Geometry: final body of the model. Coordinates: model frame, mm. Face numbers are marked on the shaded views. A direction names the side the tool comes from. Coordinates: 2 decimals unless noted, no trailing zeros. Loops run counter-clockwise (first coordinate to the right, second up) from the corner with the lowest first, then second, coordinate; pieces in that order, holes last. Notation, with made-up numbers: (45.25, 39.5) -> (72.25, 39.5) arc R10 cw to (72.25, 47.5) -> close; hole circle Ø1 at (11.5, 46). An arc over 180 degrees is marked (long way). One line per item, written item: value. Start each with the question number.
Item 1: Section query B-B on x = 44. Return loops of the section in (y, z).
Item 2: Contact query for flat-ended pins moving along their axis: pin 1 Ø5 at (y, z) = (-2, -19.5) entering from -X; pin 2 Ø10 at (x, z) = (20, 16.5) entering from -Y; pin 3 Ø3 at (x, z) = (-46.5, 14.5) entering from -Y; pin 4 Ø10 at (x, y) = (58, -6.5) entering from -Z. Output: stop coordinate, or through.
Item 3: Section query C-C on x = -35. Return loops of the section in (y, z).
Item 4: Ray query, probe 1 along Z at (x, y) = (52.5, -1); probe 2 along X at (y, z) = (-19.5, -15); probe 3 along Y at (x, z) = (-54, 0.5). Return the intervals inside material, ascending. Write a range as from..to.
Item 5: Mould query, pull axis Z, two halves, no side actions, for the marked faces 3, 4 and 5. Classes: +Z half, -Z half, draft (parallel to the pull), parting line (faces both ways), or undercut.
Item 6: Section query A-A on z = 0. Return loops of the section in (x, y).
Item 7: Set-up query: the marked faces 1 and 2. Return all of +Z, -Z, +X, -X, +Y, -Y with unobstructed straight access to the full face (end or side cutting, diameter ignored); none if empty.
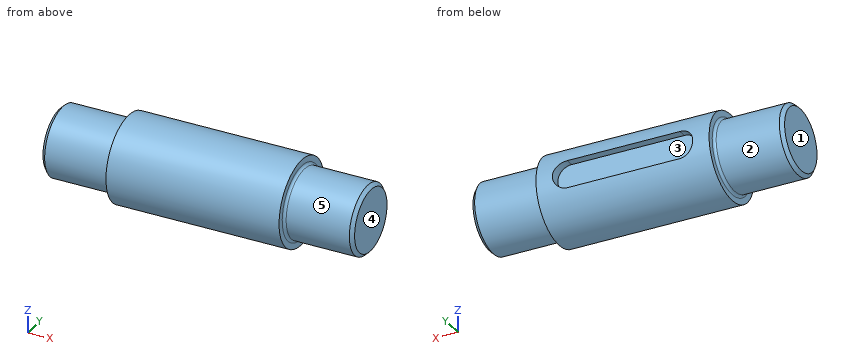
from build123d import *

# Parameters (mm, degrees)
CHANFREIN1_SIZE         = 2
ENL_V_MAT_EXTRU_1_DEPTH = 6


with BuildPart() as part:
    # Esquisse1 → Révolution1 (revolve)
    with BuildSketch(Plane(origin=(0, 0, 0), x_dir=(1, 0, 0), z_dir=(0, 1, 0)), mode=Mode.PRIVATE) as r_volution1_sk:
        with BuildLine():
            Line((-90, 0), (-90, 20))
            Line((-90, 20), (-51.5, 20))
            ThreePointArc((-51.5, 20), (-50.439339828, 20.439339828), (-50, 21.5))
            Line((-50, 21.5), (-50, 25))
            Line((-50, 25), (50, 25))
            Line((50, 25), (50, 21.5))
            ThreePointArc((50, 21.5), (50.439339828, 20.439339828), (51.5, 20))
            Line((51.5, 20), (90, 20))
            Line((90, 20), (90, 0))
            Line((90, 0), (-90, 0))
        make_face()
    revolve(r_volution1_sk.sketch.rotate(Axis((-90, 0, 0), (1, 0, 0)), 180), axis=Axis((-90, 0, 0), (1, 0, 0)))

    # Chanfrein1
    chanfrein1_edges = [part.edges().sort_by_distance(p)[0] for p in [
        (-90, 0, -20),
        (90, 0, -20),
    ]]
    chamfer(chanfrein1_edges, length=CHANFREIN1_SIZE)

    # Esquisse2 → Enlèv. mat.-Extru.1 (cut)
    with BuildSketch(Plane(origin=(0, 25, 0), x_dir=(1, 0, 0), z_dir=(0, 1, 0))):
        with BuildLine():
            Line((-32.5, 8), (32.5, 8))
            ThreePointArc((32.5, 8), (40.5, 0), (32.5, -8))
            Line((32.5, -8), (-32.5, -8))
            ThreePointArc((-32.5, -8), (-40.5, 0), (-32.5, 8))
        make_face()
    extrude(amount=-ENL_V_MAT_EXTRU_1_DEPTH, mode=Mode.SUBTRACT)


solid = part.part
Reply:
1. outline: circle Ø50 at (0, 0)
2. pin 1: stops at x = -90
2. pin 2: stops at y = -22.2
2. pin 3: stops at y = -21.35
2. pin 4: stops at z = -19.94
3. outline: (19, -7.6) -> (19, 7.6) -> (23.82, 7.6) arc R25 ccw (long way) to (23.82, -7.6) -> close
4. probe 1: z = -19.97..19.97
4. probe 2: x = -50..50
4. probe 3: y = -19.99..19.99
5. face 3: undercut
5. face 4: draft
5. face 5: parting line
6. outline: (-90, -18) -> (-88, -20) -> (-51.5, -20) arc R1.5 cw to (-50, -21.5) -> (-50, -25) -> (50, -25) -> (50, -21.5) arc R1.5 cw to (51.5, -20) -> (88, -20) -> (90, -18) -> (90, 18) -> (88, 20) -> (51.5, 20) arc R1.5 cw to (50, 21.5) -> (50, 25) -> (40.5, 25) -> (40.5, 19) -> (-40.5, 19) -> (-40.5, 25) -> (-50, 25) -> (-50, 21.5) arc R1.5 cw to (-51.5, 20) -> (-88, 20) -> (-90, 18) -> close
7. face 1: +Z, -Z, -X, +Y, -Y
7. face 2: -X
